Work out the finished part from the listing and answer in its coordinate system (mm). A direction names the side the tool comes from. Coordinates: 2 decimals unless noted, no trailing zeros. Order: outer loops, then holes, each group sorted by start corner. A loop starts at its lowest first (then second) coordinate and runs counter-clockwise, first axis right, second up. Notation, with made-up numbers: M -1.75,31 L 10.25,31 A8 ccw 10.25,45 Z; hole C -19,-9.75 d8. An arc over 180 degrees is marked long. Answer in a Markdown table with one row per item. Add a question column.
Item 1: The part is cut by section D-D (z = 541). Write down the section's boundary in (x, y).
Item 2: Consider line 1 (X direction, y = -571, z = 938.5); line 2 (X direction, y = -98, z = 543); line 3 (Z direction, x = 50.5, y = 39.5). Determine where each line is inside the solid, lowest interval first. Write a range as from..to.
Item 3: Which of the six approach directions +Z, -Z, +X, -X, +Y, -Y give full straight-line access (tool end or side, diameter ignored) to faces 1 (the face through (104.65, -421.79, 906.35)), 2 (the face through (29.58, 15.02, 47.69)), 3 (the face through (39, -439.618, 892)), 4 (the face through (39.44, -269.975, 896.57))?
Item 4: The part is cut by section C-C (x = 194). Write down the section's boundary in (y, z).
Item 5: The part is cut by section B-B (z = 807.5). State how many separate pieces and enclosed holes the cut face has, then the cut area to 3 significant figures.
Item 6: The mould has two halves that part along X. Classify faces 5 (the face through (260, -406, 894)), 6 (the face through (130, -459, 894)), 7 (the face through (39, -375, 935.48)): released by +X, released by -X, zero draft, split by the parting line, or undercut.
Item 7: Flat-ended cylindrical pins translate along their axes: pin 1 Ø4 at (y, z) = (-118, 135) entering from +X; pin 2 Ø4 at (x, y) = (43, -122) entering from -Z; pin 3 Ø12 at (x, y) = (170.5, -577) entering from +Z. Find the tip coordinate at first contact, or state that the pin passes through.
Item 8: The part is cut by section A-A (y = 0). Write down the section's boundary in (x, z), then the cut area to 3 significant figures.
from build123d import *

# Parameters (mm, degrees)
BOSS_EXTRUDE1_DEPTH = 80
SKETCH3_R           = 50
CUT_EXTRUDE1_DEPTH  = 60
SKETCH4_W           = 80
SKETCH4_H           = 25.189285717
BOSS_EXTRUDE2_DEPTH = 16
SKETCH5_W           = 80
SKETCH5_H           = 109.43946138
BOSS_EXTRUDE3_DEPTH = 16
SKETCH6_R           = 3.834610425
BOSS_EXTRUDE4_DEPTH = 78
SKETCH7_R           = 6
BOSS_EXTRUDE5_DEPTH = 135
SKETCH9_R           = 20
BOSS_EXTRUDE6_DEPTH = 50
SKETCH10_R          = 275
BOSS_EXTRUDE7_DEPTH = 130
FILLET1_R           = 40


with BuildPart() as part:
    # Sketch1 → Boss-Extrude1 (new body)
    with BuildSketch(Plane(origin=(0, 0, 0), x_dir=(0, 0, -1), z_dir=(1, 0, 0))):
        with BuildLine():
            Line((-48.50457236, 168.143707763), (-244.683369844, 111.551826897))
            Line((-244.683369844, 111.551826897), (-935.480433622, -312.64385861))
            Line((-935.480433622, -312.64385861), (-935.480433622, -439.618269219))
            Line((-935.480433622, -439.618269219), (-846.646989911, -439.618269219))
            Line((-846.646989911, -439.618269219), (-846.646989911, -379.079220955))
            Line((-846.646989911, -379.079220955), (-500.622904168, -166.597246219))
            Line((-500.622904168, -166.597246219), (0, -175))
            ThreePointArc((0, -175), (173.277449281, 24.4933781), (-48.50457236, 168.143707763))
        make_face()
    extrude(amount=BOSS_EXTRUDE1_DEPTH)

    # Sketch3 → Cut-Extrude1 (cut)
    with BuildSketch(Plane.ZY):
        Circle(SKETCH3_R)
    extrude(amount=-CUT_EXTRUDE1_DEPTH, mode=Mode.SUBTRACT)

    # Sketch4 → Boss-Extrude2 (add)
    with BuildSketch(Plane(origin=(0, 190.115415773, 116.743604378), x_dir=(1, 0, 0), z_dir=(0, 0.8521590965506677, 0.5232827860401581))):
        with Locations((40, -629.342954153)):
            Rectangle(SKETCH4_W, SKETCH4_H)
    extrude(amount=BOSS_EXTRUDE2_DEPTH)

    # Sketch5 → Boss-Extrude3 (add)
    with BuildSketch(Plane(origin=(0, 190.115415773, 116.743604378), x_dir=(1, 0, 0), z_dir=(0, 0.8521590965506677, 0.5232827860401581))):
        with Locations((40, -906.059579837)):
            Rectangle(SKETCH5_W, SKETCH5_H)
    extrude(amount=BOSS_EXTRUDE3_DEPTH)

    # Sketch6 → Boss-Extrude4 (add)
    with BuildSketch(Plane(origin=(0, -335.914894228, 547.032962711), x_dir=(1, 0, 0), z_dir=(0, -0.5232827860401581, 0.8521590965506677))):
        with Locations(Location((22.669741736, 230.944821583, 0), (0, 0, 90))):
            Circle(SKETCH6_R)
        with Locations(Location((57.330258264, 230.944821583, 0), (0, 0, 90))):
            Circle(SKETCH6_R)
    extrude(amount=BOSS_EXTRUDE4_DEPTH)

    # Sketch7 → Boss-Extrude5 (add)
    with BuildSketch(Plane(origin=(0, -376.730951539, 613.501372242), x_dir=(1, 0, 0), z_dir=(0, -0.5232827860401581, 0.8521590965506677))):
        with Locations(Location((22.669741736, 230.944821583, 0), (0, 0, 270))):
            Circle(SKETCH7_R)
        with Locations(Location((57.330258264, 230.944821583, 0), (0, 0, 270))):
            Circle(SKETCH7_R)
    extrude(amount=BOSS_EXTRUDE5_DEPTH)

    # Sketch9 → Boss-Extrude6 (add)
    with BuildSketch(Plane(origin=(80, 0, 0), x_dir=(0, 0, -1), z_dir=(1, 0, 0))):
        with Locations((-890.480433622, -409.618269219)):
            Circle(SKETCH9_R)
    extrude(amount=BOSS_EXTRUDE6_DEPTH)

    # Sketch10 → Boss-Extrude7 (add)
    with BuildSketch(Plane(origin=(130, 0, 0), x_dir=(0, 0, -1), z_dir=(1, 0, 0))):
        with Locations((-890.480433622, -409.618269219)):
            Circle(SKETCH10_R)
    extrude(amount=BOSS_EXTRUDE7_DEPTH)

    # Fillet1
    fillet1_edges = [part.edges().sort_by_distance(p)[0] for p in [
        (130, -409.618269219, 1165.480433622),
        (260, -409.618269219, 1165.480433622),
    ]]
    fillet(fillet1_edges, radius=FILLET1_R)


solid = part.part
Reply:
| question | item | result |
|---|---|---|
| 1 | outline | M 0,-191.39 L 80,-191.39 L 80,-70.41 L 0,-70.41 Z |
| 2 | line 1 | x = 130..260 |
| 2 | line 2 | x = 0..80 |
| 2 | line 3 | z = -170.48..-30.66, 30.66..362.02 |
| 3 | face 1 | none |
| 3 | face 2 | -X |
| 3 | face 3 | +Z, -Z, -X, -Y |
| 3 | face 4 | +Z, -X, +Y |
| 4 | outline | C -409.62,890.48 d550 |
| 5 | separate pieces | 4 |
| 5 | enclosed holes | 0 |
| 5 | area | 76,700 mm2 |
| 6 | face 5 | released by +X |
| 6 | face 6 | undercut |
| 6 | face 7 | zero draft |
| 7 | pin 1 | stops at x = 80 |
| 7 | pin 2 | stops at z = -127.38 |
| 7 | pin 3 | stops at z = 1113.15 |
| 8 | outline | M 0,-175 L 80,-175 L 80,426.34 L 0,426.34 L 0,50 L 60,50 L 60,-50 L 0,-50 Z |
| 8 | area | 42,100 mm2 |
